```python
from build123d import *

# Parameters (mm, degrees)
SKETCH1_R           = 4
BOSS_EXTRUDE1_DEPTH = 6


with BuildPart() as part:
    # Sketch1 → Boss-Extrude1 (new body)
    with BuildSketch(Plane.XY):
        with BuildLine():
            Line((-37.787642532, 307.932576411), (-123.887642532, 307.932576411))
            Line((-123.887642532, 307.932576411), (-137.545094515, 300.047977161))
            ThreePointArc((-137.545094515, 300.047977161), (-141.205529316, 296.38770347), (-142.545348637, 291.387576411))
            Line((-142.545348637, 291.387576411), (-142.545348637, 259.477576411))
            ThreePointArc((-142.545348637, 259.477576411), (-141.205529316, 254.477449351), (-137.545094515, 250.817175661))
            Line((-137.545094515, 250.817175661), (-123.887642532, 242.932576411))
            Line((-123.887642532, 242.932576411), (-37.787642532, 242.932576411))
            Line((-37.787642532, 242.932576411), (-37.787642532, 307.932576411))
        make_face()
        with Locations((-118.785348637, 275.432576411)):
            Circle(SKETCH1_R, mode=Mode.SUBTRACT)
    extrude(amount=BOSS_EXTRUDE1_DEPTH)


solid = part.part
```
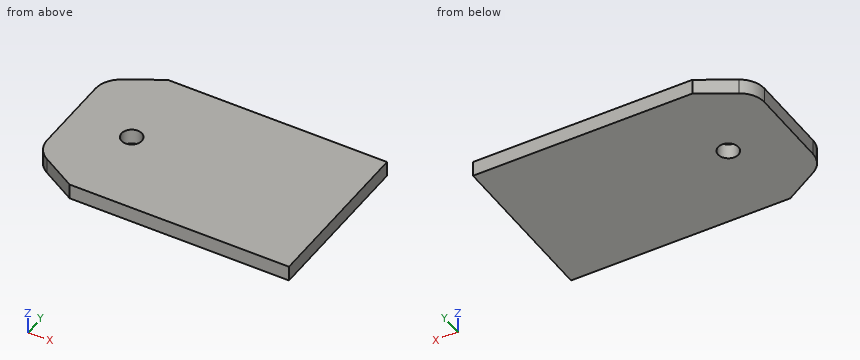
Verification items for the finished model (mm, model axes). Give positions to 0.01 mm unless a question says otherwise; leave off trailing zeros. Order: outer loops, then holes, each group sorted by start corner. A loop starts at its lowest first (then second) coordinate and runs counter-clockwise, first axis right, second up. Notation, with made-up numbers: M 88,25 L 108,25 A28 ccw 108,51 Z; hole C -17.75,56.5 d6. An arc over 180 degrees is marked long. Return JSON: item names as keys, results as strings. Group by question number.
1) Section check D-D on y = 297. Record the cut outline in (x, z), and give its area (3 significant figures).
2) Section check A-A on x = -118. Record the cut outline in (y, z).
3) Section check B-B on y = 276.5. Record the cut outline in (x, z), and give its area (3 significant figures).
4) Scan lines: line 1 (X direction, y = 275, z = 2.85); line 2 (X direction, y = 276.5, z = 2.65); line 3 (Y direction, x = -122, z = 2.95). Record each from-to range of solid material in increasing order.
5) Section check C-C on z = 2.6. Record the cut outline in (x, y).
Answer block:
{
 "1": {"outline": "M -140.82,0 L -37.79,0 L -37.79,6 L -140.82,6 Z", "area": "618 mm^2"},
 "2": {"outline": "M 242.93,0 L 271.51,0 L 271.51,6 L 242.93,6 Z; M 279.35,0 L 307.93,0 L 307.93,6 L 279.35,6 Z"},
 "3": {"outline": "M -142.55,0 L -122.64,0 L -122.64,6 L -142.55,6 Z; M -114.93,0 L -37.79,0 L -37.79,6 L -114.93,6 Z", "area": "582 mm^2"},
 "4": {"line 1": "x = -142.55 to -122.76, -114.81 to -37.79", "line 2": "x = -142.55 to -122.64, -114.93 to -37.79", "line 3": "y = 242.93 to 273.05, 277.81 to 307.93"},
 "5": {"outline": "M -142.55,259.48 A10 ccw -137.55,250.82 L -123.89,242.93 L -37.79,242.93 L -37.79,307.93 L -123.89,307.93 L -137.55,300.05 A10 ccw -142.55,291.39 Z; hole C -118.79,275.43 d8"}
}
